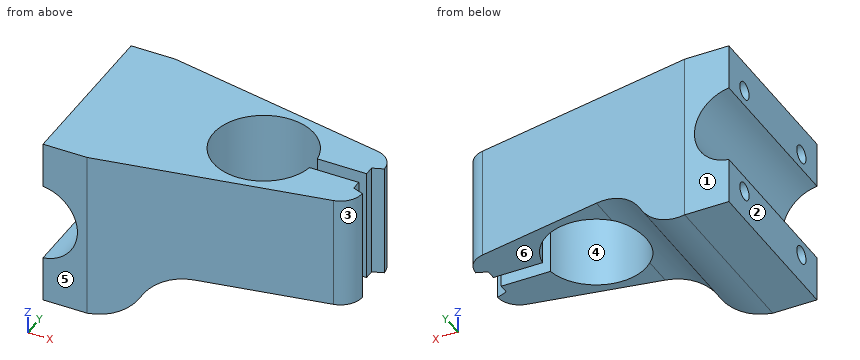
from build123d import *

# Parameters (mm, degrees)
F1_DEPTH = 24
F3_DEPTH = 48
F5_DEPTH = 48
F7_D     = 5
F7_DEPTH = 12
F7_TIP   = 1.5021515476


with BuildPart() as f1:
    # F0 (on Top) → F1 (new body, symmetric)
    with BuildSketch(Plane.XY):
        with BuildLine():
            Line((-24.6308942474, 24), (-37.1308942474, 24))
            Line((-37.1308942474, 24), (-37.1308942474, 0))
            Line((-37.1308942474, 0), (-37.1308942474, -24))
            Line((-37.1308942474, -24), (-24.6308942474, -24))
            Line((-24.6308942474, -24), (38.8693180593, -12.0302915725))
            ThreePointArc((38.8693180593, -12.0302915725), (42.4565903396, -9.9167044), (43.8691057526, -6))
            Line((43.8691057526, -6), (40.8691057526, -4.875))
            Line((40.8691057526, -4.875), (40.8691057526, -2.125))
            Line((40.8691057526, -2.125), (26.9597719895, -2.125))
            ThreePointArc((26.9597719895, -2.125), (-1.3808942474, 0), (26.9597719895, 2.125))
            Line((26.9597719895, 2.125), (40.8691057526, 2.125))
            Line((40.8691057526, 2.125), (40.8691057526, 4.875))
            Line((40.8691057526, 4.875), (43.8691057526, 6))
            ThreePointArc((43.8691057526, 6), (42.4565903396, 9.9167044), (38.8693180593, 12.0302915725))
            Line((38.8693180593, 12.0302915725), (-24.6308942474, 24))
        make_face()
    extrude(amount=F1_DEPTH, both=True)

    # F2 (on face) → F3 (cut, through all)
    with BuildSketch(Plane.XZ.offset(24)):
        with BuildLine():
            ThreePointArc((-10.7744877868, -16), (-16.6308942474, -21.8564064606), (-24.6308942474, -24))
            Line((-24.6308942474, -24), (48.1037423015, -24))
            Line((48.1037423015, -24), (48.1037423015, -8))
            Line((48.1037423015, -8), (3.0819186737, -8))
            ThreePointArc((3.0819186737, -8), (-4.9180813263, -10.1435935394), (-10.7744877868, -16))
        make_face()
    extrude(amount=-F3_DEPTH, mode=Mode.SUBTRACT)

    # F4 (on face) → F5 (cut, through all)
    with BuildSketch(Plane.XZ.offset(24)):
        with BuildLine():
            Line((-37.1308942474, 11.0286558564), (-37.1308942474, -11.0286558564))
            ThreePointArc((-37.1308942474, -11.0286558564), (-27.3808942474, 0), (-37.1308942474, 11.0286558564))
        make_face()
    extrude(amount=-F5_DEPTH, mode=Mode.SUBTRACT)

    # F7
    with Locations(Plane(origin=(-37.1308942474, 0, 0), x_dir=(0, -1, 0), z_dir=(-1, 0, 0))):
        with Locations((-15.5, 15.5), (15.5, 15.5), (15.5, -15.5), (-15.5, -15.5)):
            Hole(F7_D / 2, depth=F7_DEPTH)
            with Locations((0, 0, -(F7_DEPTH + F7_TIP / 2))):  # 118° drill point
                Cone(0, F7_D / 2, F7_TIP, mode=Mode.SUBTRACT)


solid = f1.part
Part model, mm, in its own coordinate system. Face numbers are marked on the shaded views. A direction names the side the tool comes from. Coordinates: 2 decimals unless noted, no trailing zeros. Order: outer loops, then holes, each group sorted by start corner. A loop starts at its lowest first (then second) coordinate and runs counter-clockwise, first axis right, second up. Notation, with made-up numbers: (-27, -13.75) - (-7, -13.75) arc R14 ccw to (-7, -7.75) - close; hole circle Ø10 at (68.25, -15). An arc over 180 degrees is marked (long way). Use CSV: the item, a comma, the result in double quotes.
Item 1: Saw through at A-A on x = 11. Give the cut face in (y, z), and give its area (3 significant figures).
Solved:
outline,"(-17.28, -8) - (-14.13, -8) - (-14.13, 24) - (-17.28, 24) - close; (14.13, -8) - (17.28, -8) - (17.28, 24) - (14.13, 24) - close"
area,"202 mm²"
Item 2: Drop flat-ended pins along their axis: P1, Ø4, axis at x = 34.5, z = 9, coming from the -Y side; P2, Ø5, axis at x = 4, z = 4.5, coming from the +Y side; P3, Ø8, axis at y = 15.5, z = -15.5, coming from the -X side; P4, Ø5, axis at x = 31.5, y = 12.5, coming from the -Z side. Give the stop position or say it passes through.
Solved:
P1,"stops at y = -13.23"
P2,"stops at y = 19.07"
P3,"stops at x = -37.13"
P4,"stops at z = -8"
Item 3: Saw through at B-B on z = 12. Give the cut face in (x, y) (3 decimals).
Solved:
outline,"(-37.131, -24) - (-24.631, -24) - (38.869, -12.03) arc R6.136 ccw to (43.869, -6) - (40.869, -4.875) - (40.869, -2.125) - (26.96, -2.125) arc R14.25 cw (long way) to (26.96, 2.125) - (40.869, 2.125) - (40.869, 4.875) - (43.869, 6) arc R6.136 ccw to (38.869, 12.03) - (-24.631, 24) - (-37.131, 24) - close"
Item 4: Mould opens along Y. For the marked faces 1, 2, 3 and 4 say: +Y half, -Y half, draft (parallel to the pull), parting line (faces both ways), or undercut.
Solved:
face 1,"+Y half"
face 2,"draft"
face 3,"-Y half"
face 4,"undercut"
Item 5: Probe probe 1 along Y at (x, z) = (-30, -15.5); probe 2 along Z at (x, y) = (-31, -15.5); probe 3 along Y at (x, z) = (-30, 15). List the from-to ranges inside material, lowest first.
Solved:
probe 1,"y = -24 to -18, -13 to 13, 18 to 24"
probe 2,"z = -24 to -18, -13 to -8.21, 8.21 to 13, 18 to 24"
probe 3,"y = -24 to -17.95, -13.05 to 13.05, 17.95 to 24"
Item 6: Saw through at C-C on x = 19.5. Give the cut face in (y, z), and give its area (3 significant figures).
Solved:
outline,"(-15.68, -8) - (-12.61, -8) - (-12.61, 24) - (-15.68, 24) - close; (12.61, -8) - (15.68, -8) - (15.68, 24) - (12.61, 24) - close"
area,"196 mm²"
Item 7: Saw through at D-D on x = -18.5. Give the cut face in (y, z), and give its area (3 significant figures).
Solved:
outline,"(-22.84, -22.78) - (22.84, -22.78) - (22.84, 24) - (-22.84, 24) - close"
area,"2,140 mm²"
Item 8: 3-axis set-ups, long thin cutter, end or side, ignore diameter. For the marked faces 5 and 6: which of +Z, -Z, +X, -X, +Y, -Y reach the whole face in a straight line?
Solved:
face 5,"+Z, -Z, +X, -X, -Y"
face 6,"-Z, +X, +Y, -Y"
